Work out the finished part from the listing and answer in its coordinate system (mm). A direction names the side the tool comes from. Coordinates: 2 decimals unless noted, no trailing zeros. Loops run counter-clockwise (first coordinate to the right, second up) from the corner with the lowest first, then second, coordinate; pieces in that order, holes last. Notation, with made-up numbers: (-31.5, 73) -> (-11.5, 73) arc R12 cw to (-11.5, 85) -> close; hole circle Ø10 at (2, 5). An arc over 180 degrees is marked (long way). Answer as CSV lines item,"result".
```python
from build123d import *

# Parameters (mm, degrees)
F0_R     = 33.75
F0_R_2   = 25.75
F1_DEPTH = 15
F3_DEPTH = 20
F4_COUNT = 6
F6_R     = 1.35
F7_DEPTH = 40
F9_COUNT = 6


with BuildPart() as f1:
    # F0 (on Top) → F1 (new body)
    with BuildSketch(Plane.XY):
        Circle(F0_R)
        Circle(F0_R_2, mode=Mode.SUBTRACT)
    extrude(amount=F1_DEPTH)


with BuildPart() as f3:
    # F2 (on face) → F3 (new body)
    with BuildSketch(Plane.XY.offset(15)):
        Polygon((-26.575, -1.833087), (-26.575, 1.833087), (-29.75, 3.666174), (-32.925, 1.833087), (-32.925, -1.833087), (-29.75, -3.666174), align=None)
    extrude(amount=-F3_DEPTH)


with BuildPart() as f4_1:
    # F4: instance of F3
    add(f3.part.rotate(Axis((0, 0, 15), (0, 0, 1)), 1 * 360 / F4_COUNT))


with BuildPart() as f4_2:
    # F4: instance of F3
    add(f3.part.rotate(Axis((0, 0, 15), (0, 0, 1)), 2 * 360 / F4_COUNT))


with BuildPart() as f4_3:
    # F4: instance of F3
    add(f3.part.rotate(Axis((0, 0, 15), (0, 0, 1)), 3 * 360 / F4_COUNT))


with BuildPart() as f4_4:
    # F4: instance of F3
    add(f3.part.rotate(Axis((0, 0, 15), (0, 0, 1)), 4 * 360 / F4_COUNT))


with BuildPart() as f4_5:
    # F4: instance of F3
    add(f3.part.rotate(Axis((0, 0, 15), (0, 0, 1)), 5 * 360 / F4_COUNT))


with BuildPart() as f1_1:
    add(f1.part)

    # F5: cut F4_1, F3, F4_2, F4_3, F4_4, F4_5
    add(f4_1.part, mode=Mode.SUBTRACT)
    add(f3.part, mode=Mode.SUBTRACT)
    add(f4_2.part, mode=Mode.SUBTRACT)
    add(f4_3.part, mode=Mode.SUBTRACT)
    add(f4_4.part, mode=Mode.SUBTRACT)
    add(f4_5.part, mode=Mode.SUBTRACT)


with BuildPart() as f7:
    # F6 (on Front) → F7 (new body)
    with BuildSketch(Plane.XZ):
        with Locations((0, 7.524926)):
            Circle(F6_R)
    extrude(amount=F7_DEPTH)


with BuildPart() as f7_1:
    # F8: moved
    add(f7.part.moved(Location((0, -26, 0))))


with BuildPart() as f9_1:
    # F9: instance of F7
    add(f7_1.part.rotate(Axis((0, 0, 15), (0, 0, 1)), 1 * 360 / F9_COUNT))


with BuildPart() as f9_2:
    # F9: instance of F7
    add(f7_1.part.rotate(Axis((0, 0, 15), (0, 0, 1)), 2 * 360 / F9_COUNT))


with BuildPart() as f9_3:
    # F9: instance of F7
    add(f7_1.part.rotate(Axis((0, 0, 15), (0, 0, 1)), 3 * 360 / F9_COUNT))


with BuildPart() as f9_4:
    # F9: instance of F7
    add(f7_1.part.rotate(Axis((0, 0, 15), (0, 0, 1)), 4 * 360 / F9_COUNT))


with BuildPart() as f9_5:
    # F9: instance of F7
    add(f7_1.part.rotate(Axis((0, 0, 15), (0, 0, 1)), 5 * 360 / F9_COUNT))


with BuildPart() as f1_2:
    add(f1_1.part)

    # F10: cut F7, F9_1, F9_2, F9_3, F9_4, F9_5
    add(f7_1.part, mode=Mode.SUBTRACT)
    add(f9_1.part, mode=Mode.SUBTRACT)
    add(f9_2.part, mode=Mode.SUBTRACT)
    add(f9_3.part, mode=Mode.SUBTRACT)
    add(f9_4.part, mode=Mode.SUBTRACT)
    add(f9_5.part, mode=Mode.SUBTRACT)


solid = f1_2.part
```
(1) Flat-ended cylindrical pins translate along their axes: pin 1 Ø3 at (x, z) = (1, 6) entering from -Y; pin 2 Ø3 at (y, z) = (-25, 5) entering from -X; pin 3 Ø1.4 at (x, z) = (0, 8) entering from -Y; pin 4 Ø6 at (y, z) = (-9, 6.5) entering from -X. Find the tip coordinate at first contact, or state that the pin passes through.
Computed values:
pin 1,"y = -33.75"
pin 2,"x = -24.22"
pin 3,"y = -26"
pin 4,"x = -33.21"
(2) Which of the six approach directions +Z, -Z, +X, -X, +Y, -Y give full straight-line access (tool end or side, diameter ignored) to faces 1 (the face through (16.44, 23, 7.6)), 2 (the face through (-22.53, -12.98, 7.54))?
Computed values:
face 1,"+Z, -Z"
face 2,"none"
(3) For a pull along Y with two mould halves and no side action, classify faces 3 (the face through (0, 26, 8)), 4 (the face through (32.925, 0, 8)), 5 (the face through (-0.176, -29.821, 8.863)) as pulls with the +Y half, pulls with the -Y half, needs draft (parallel to the pull), parting line crosses it, or undercut.
Computed values:
face 3,"pulls with the +Y half"
face 4,"undercut"
face 5,"needs draft"
(4) A cutting plane is placed at D-D, the plane x = 14. Write down the section's boundary in (y, z), and give its area (3 significant figures).
Computed values:
outline,"(-30.71, 0) -> (-28.93, 0) -> (-28.93, 15) -> (-30.71, 15) -> close; (-22.6, 0) -> (-21.61, 0) -> (-21.61, 15) -> (-22.6, 15) -> close; (21.61, 0) -> (22.6, 0) -> (22.6, 15) -> (21.61, 15) -> close; (28.93, 0) -> (30.71, 0) -> (30.71, 15) -> (28.93, 15) -> close"
area,"83.3 mm2"
(5) A cutting plane is placed at B-B, the plane y = 0. Write down the section's boundary in (x, z) (3 decimals).
Computed values:
outline,"(-33.75, 0) -> (-32.925, 0) -> (-32.925, 15) -> (-33.75, 15) -> close; (-26.575, 0) -> (-25.75, 0) -> (-25.75, 15) -> (-26.575, 15) -> close; (25.75, 0) -> (26.575, 0) -> (26.575, 15) -> (25.75, 15) -> close; (32.925, 0) -> (33.75, 0) -> (33.75, 15) -> (32.925, 15) -> close"
(6) A cutting plane is placed at C-C, the plane y = 7. Write down the section's boundary in (x, z), and give its area (3 significant figures).
Computed values:
outline,"(-33.02, 0) -> (-24.78, 0) -> (-24.78, 15) -> (-33.02, 15) -> close; (24.78, 0) -> (33.02, 0) -> (33.02, 15) -> (24.78, 15) -> close"
area,"247 mm2"
(7) Consider line 1 along Z through (x, y) = (0, -29.25); line 2 along X through (y, z) = (1, 11) (3 decimals); line 3 along Y through (x, z) = (17, 5.75). Determine where each line is inside the solid, lowest interval first.
Computed values:
line 1,"0 to 6.17, 8.87 to 15"
line 2,"-33.735 to -32.925, -26.575 to -25.731, 25.731 to 26.575, 32.925 to 33.735"
line 3,"-29.16 to -28.2, -23.32 to -19.34, 19.34 to 23.32, 28.2 to 29.16"
(8) A cutting plane is placed at A-A, the plane x = 0. Write down the section's boundary in (y, z), and give its area (3 significant figures).
Computed values:
outline,"(-33.75, 0) -> (-25.75, 0) -> (-25.75, 15) -> (-33.75, 15) -> (-33.75, 8.87) -> (-26, 8.87) -> (-26, 6.17) -> (-33.75, 6.17) -> close; (25.75, 0) -> (33.75, 0) -> (33.75, 6.17) -> (26, 6.17) -> (26, 8.87) -> (33.75, 8.87) -> (33.75, 15) -> (25.75, 15) -> close"
area,"198 mm2"
